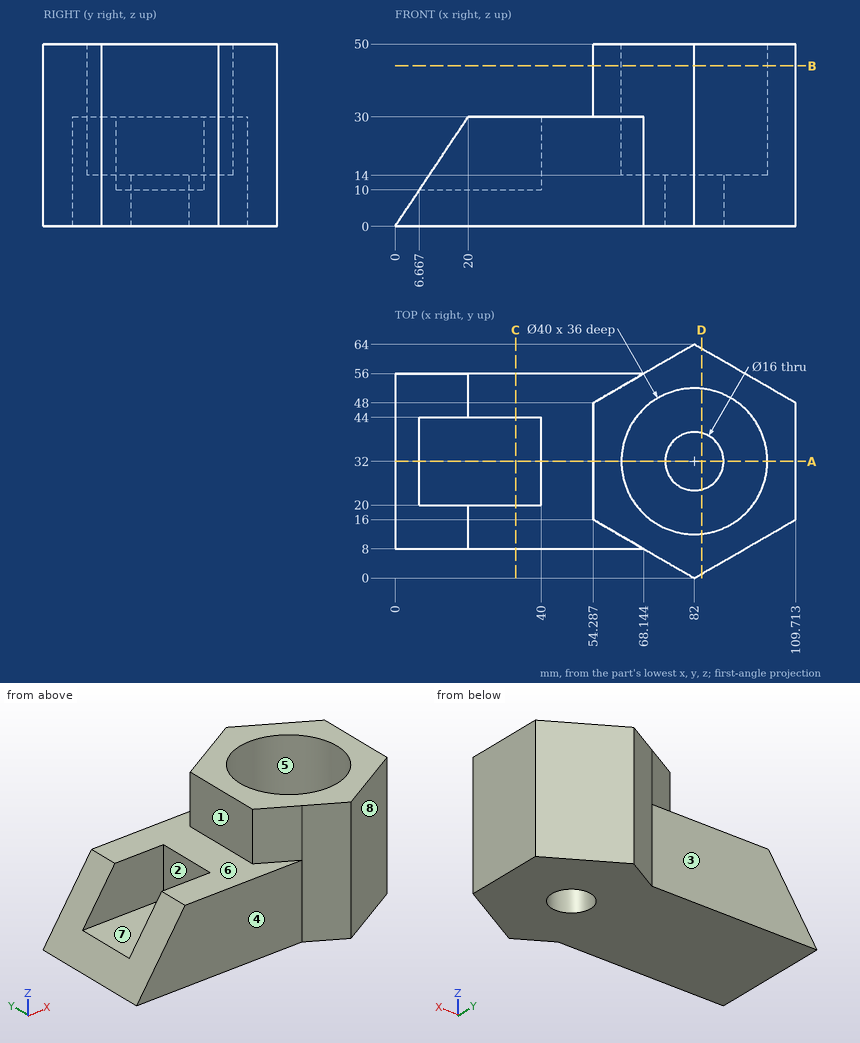
Could you check a few things on this drawing? It's one solid part, dimensions in mm from its lowest x, y, z. A direction names the side the tool comes from. Round coordinates to 2 decimals unless told otherwise and drop trailing zeros. Loops run counter-clockwise (first coordinate to the right, second up) from the corner with the lowest first, then second, coordinate; pieces in that order, holes last.
Q1. Thinking about a two-plate mould opening in Y: for the marked faces 6, 7 and 8, which applies, pulls with the +Y half, pulls with the -Y half, needs draft (parallel to the pull), parting line crosses it, or undercut?
Q2. I want a section at B-B (z = 44). Write out the boundary of the cut face in (x, y), and give its area (3 significant figures).
Q3. Please list where these lines run through material, in increasing order: L1, parallel to Y at x = 82, z = 5.5; L2, parallel to Y at x = 82, z = 23; L3, parallel to Z at x = 26, y = 45.
Q4. For P1, Ø19, axis at x = 23, y = 31, coming from the +Z side; P2, Ø10, axis at y = 56.5, z = 36, coming from the -X side; P3, Ø1.5, axis at y = 56, z = 21.5, coming from the +X side (1 decimal), each with a flat end and sliding along its axis, tell me the tip position at first contact or that it passes through.
Q5. I want a section at A-A (y = 32). Write out the boundary of the cut face in (x, z).
Q6. I want a section at C-C (x = 33). Write out the boundary of the cut face in (y, z), and give its area (3 significant figures).
Q7. I want a section at D-D (x = 84). Write out the boundary of the cut face in (y, z) (1 decimal), and give its area (4 significant figures).
Q8. On a 3-axis mill with a long thin cutter (end or side, diameter ignored), from which of +Z, -Z, +X, -X, +Y, -Y can I reach the whole of each face in a straight line? I mean the marked faces 1, 2, 3, 4 and 5. Say none if no direction works.
Answer below:
1. face 6: needs draft
1. face 7: undercut
1. face 8: pulls with the -Y half
2. outline: (54.29, 16) - (82, 0) - (109.71, 16) - (109.71, 48) - (82, 64) - (54.29, 48) - close; hole circle Ø40 at (82, 32)
2. area: 1,400 mm2
3. L1: y = 0 to 24, 40 to 64
3. L2: y = 0 to 12, 52 to 64
3. L3: z = 0 to 30
4. P1: stops at z = 10
4. P2: stops at x = 60.35
4. P3: stops at x = 97.2
5. outline: (0, 0) - (74, 0) - (74, 14) - (62, 14) - (62, 50) - (54.29, 50) - (54.29, 30) - (40, 30) - (40, 10) - (6.67, 10) - close; (90, 0) - (109.71, 0) - (109.71, 50) - (102, 50) - (102, 14) - (90, 14) - close
6. outline: (8, 0) - (56, 0) - (56, 30) - (44, 30) - (44, 10) - (20, 10) - (20, 30) - (8, 30) - close
6. area: 960 mm2
7. outline: (1.2, 0) - (24.3, 0) - (24.3, 14) - (12.1, 14) - (12.1, 50) - (1.2, 50) - close; (39.7, 0) - (62.8, 0) - (62.8, 50) - (51.9, 50) - (51.9, 14) - (39.7, 14) - close
7. area: 1,435 mm2
8. face 1: +Z, -X, +Y, -Y
8. face 2: +Z, -X
8. face 3: +Z, -Z, -X, +Y
8. face 4: +Z, -Z, -X, -Y
8. face 5: +Z
